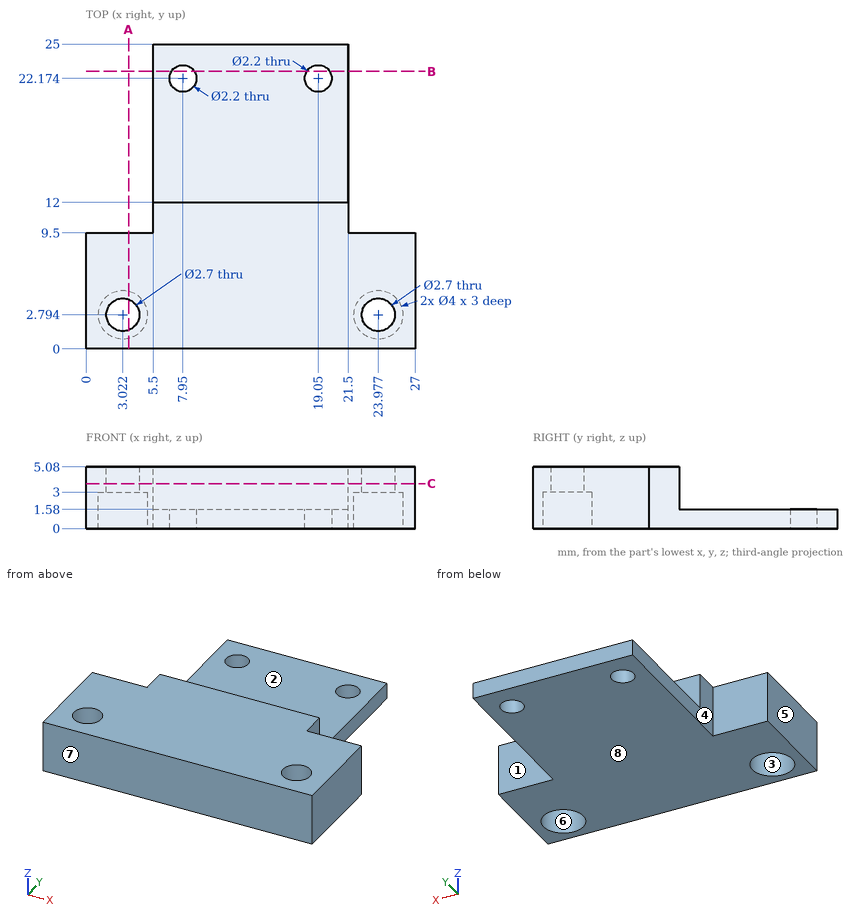
For this review, use the dimensioned drawing (mm, ordinates from the lowest corner) and the shaded views. A direction names the side the tool comes from. Give positions to 0.01 mm unless a question says otherwise; leave off trailing zeros. Order: outer loops, then holes, each group sorted by start corner. A loop starts at its lowest first (then second) coordinate and runs counter-clockwise, first axis right, second up.
1) Take a section at C-C (z = 3.7). State how many separate pieces and enclosed holes the cut face has, then the cut area to 3 significant figures.
2) Insertion check: pin 1 (1 mm diameter, centred on y = 12, z = 2.5, fed in from +X); pin 2 (1.2 mm diameter, centred on x = 24, y = 2, fed in from -Z); pin 3 (3.5 mm diameter, centred on x = 3.02, y = 2.79, fed in from +Z); pin 4 (1.6 mm diameter, centred on x = 23.98, y = 2.79, fed in from -Z) (3 decimals). Each pin has a flat end and moves straight along its axis. Give the tip position at first contact, or say it passes through.
3) Wall thickness on line 1 (Y direction, x = 6.5, z = 3.85); line 2 (Y direction, x = 5.25, z = 0.75); line 3 (Y direction, x = 2, z = 2.45) (1 decimal): over which ranges is each line inside the solid? List them lowest first.
4) For the marked faces 1, 2, 3, 4 and 5, list the 3-axis set-ups (+Z, -Z, +X, -X, +Y, -Y) from which the entire face can be reached by the end or side of a thin tool; tool diameter is ignored.
5) The part is to be moulded in two halves that separate along Y. For the marked faces 6, 7 and 8, say which applies: released by +Y, released by -Y, zero draft, split by the parting line, or undercut.
6) Take a section at B-B (y = 22.75). Give the boundary of the cut face in (x, z).
7) Take a section at A-A (x = 3.5). Give the boundary of the cut face in (y, z).
Derived:
1. separate pieces: 1
1. enclosed holes: 2
1. area: 285 mm2
2. pin 1: stops at x = 21.5
2. pin 2: stops at z = 3
2. pin 3: stops at z = 5.08
2. pin 4: passes through
3. line 1: y = 0 to 12
3. line 2: y = 0 to 9.5
3. line 3: y = 0 to 1.1, 4.5 to 9.5
4. face 1: +Z, -Z, +X, +Y
4. face 2: +Z, +X, -X, +Y
4. face 3: -Z
4. face 4: +Z, -Z, -X, +Y
4. face 5: +Z, -Z, -X, +Y, -Y
5. face 6: undercut
5. face 7: released by -Y
5. face 8: zero draft
6. outline: (5.5, 0) - (7.01, 0) - (7.01, 1.58) - (5.5, 1.58) - close; (8.89, 0) - (18.11, 0) - (18.11, 1.58) - (8.89, 1.58) - close; (19.99, 0) - (21.5, 0) - (21.5, 1.58) - (19.99, 1.58) - close
7. outline: (0, 0) - (0.85, 0) - (0.85, 3) - (1.53, 3) - (1.53, 5.08) - (0, 5.08) - close; (4.06, 3) - (4.74, 3) - (4.74, 0) - (9.5, 0) - (9.5, 5.08) - (4.06, 5.08) - close
